Answer from the drawing. Dimensions are ordinates in mm from the lowest x, y and z of the part. A direction names the side the tool comes from. Give positions to 0.01 mm unless a question says otherwise; leave off trailing zeros. Loops run counter-clockwise (first coordinate to the right, second up) from the corner with the lowest first, then second, coordinate; pieces in that order, holes last. Notation, with made-up numbers: (44, 20) -> (85, 20) arc R28 cw to (85, 44) -> close; hole circle Ø5 at (71.25, 24). An arc over 180 degrees is marked (long way). Write each question's results on one line, items separated by ' | '. Start each with the question number.
Item 1: Section A-A on x = 3 is taken. Write down the section's boundary in (y, z), and give its area (3 significant figures).
Item 2: Each of these flat-tipped pins is pushed along its axis until it touches: P1, Ø3, axis at y = 3.5, z = 8, coming from the -X side; P2, Ø3, axis at x = 9, z = 4, coming from the +Y side; P3, Ø2, axis at x = 5, y = 3, coming from the -Z side. Where does it stop, or does it pass through?
Item 3: Section B-B on z = 9.75 is taken. Write down the section's boundary in (x, y), and give its area (4 significant figures).
Item 4: Section C-C on y = 4.7 is taken. Write down the section's boundary in (x, z), and give its area (4 significant figures).
Item 5: Section D-D on x = 8.5 is taken. Write down the section's boundary in (y, z), and give its area (3 significant figures).
Item 6: Find the intervals of material crossed by line 1 (Y direction, x = 11.25, z = 3.5); line 2 (Z direction, x = 5.5, y = 2.9); line 3 (X direction, y = 3.3, z = 8.75), in increasing order.
Item 7: Which of the six approach directions +Z, -Z, +X, -X, +Y, -Y give full straight-line access (tool end or side, diameter ignored) to the marked faces 1, 2 and 3?
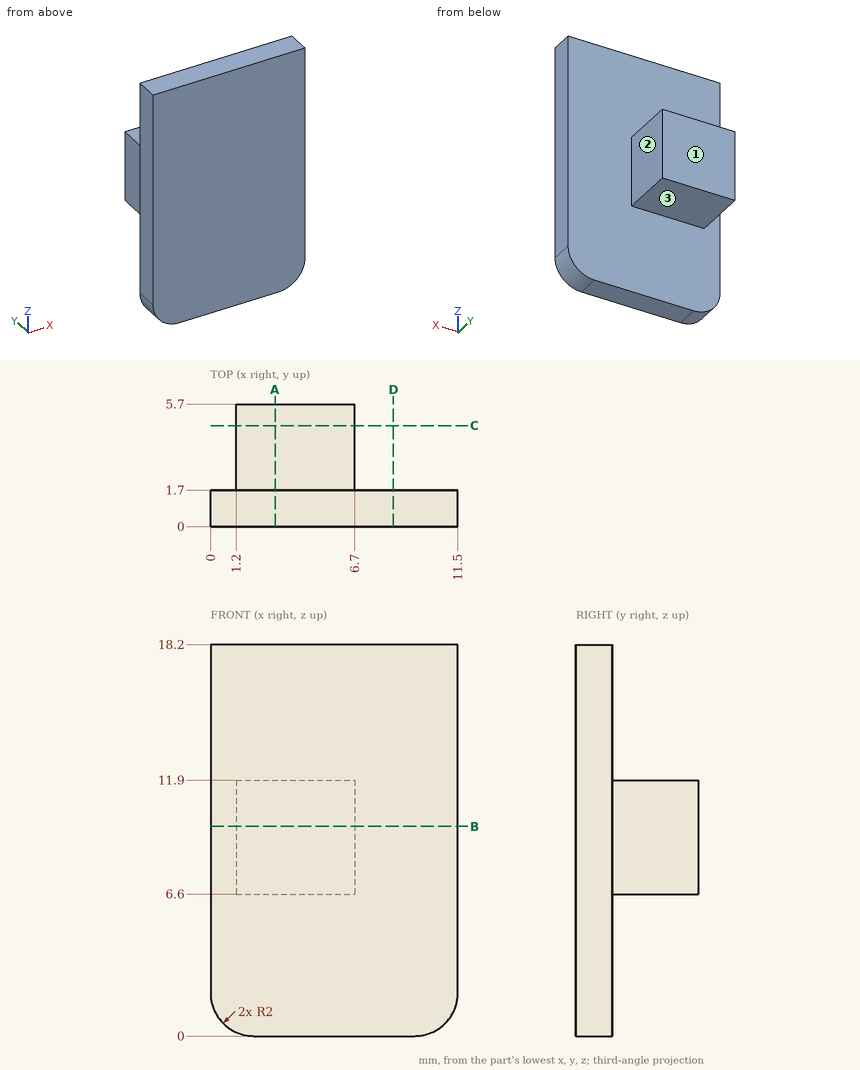
Findings:
1) outline: (0, 0) -> (1.7, 0) -> (1.7, 6.6) -> (5.7, 6.6) -> (5.7, 11.9) -> (1.7, 11.9) -> (1.7, 18.2) -> (0, 18.2) -> close | area: 52.1 mm2
2) P1: x = 1.2 | P2: y = 1.7 | P3: z = 6.6
3) outline: (0, 0) -> (11.5, 0) -> (11.5, 1.7) -> (6.7, 1.7) -> (6.7, 5.7) -> (1.2, 5.7) -> (1.2, 1.7) -> (0, 1.7) -> close | area: 41.55 mm2
4) outline: (1.2, 6.6) -> (6.7, 6.6) -> (6.7, 11.9) -> (1.2, 11.9) -> close | area: 29.15 mm2
5) outline: (0, 0) -> (1.7, 0) -> (1.7, 18.2) -> (0, 18.2) -> close | area: 30.9 mm2
6) line 1: 0 to 1.7 | line 2: 6.6 to 11.9 | line 3: 1.2 to 6.7
7) face 1: +Z, -Z, +X, -X, +Y | face 2: +Z, -Z, +X, +Y | face 3: -Z, +X, -X, +Y
